Could you check a few things on this drawing? It's one solid part, dimensions in mm from its lowest x, y, z. A direction names the side the tool comes from. Give positions to 0.01 mm unless a question says otherwise; leave off trailing zeros. Loops run counter-clockwise (first coordinate to the right, second up) from the corner with the lowest first, then second, coordinate; pieces in that order, holes last. Notation, with made-up numbers: M -17,20.5 L 3,20.5 A22 ccw 3,37.5 Z; hole C 58.25,6.25 d3. An arc over 180 degrees is marked long. Answer as CSV lines item,"result". Start each with the question number.
Item 1: Will these pins go through, and if not, where does the flat tip stop? P1, Ø5, axis at x = 364.5, z = 446.5, coming from the +Y side; P2, Ø10, axis at x = 457.5, y = 46.5, coming from the +Z side; P3, Ø2, axis at y = 214.5, z = 768, coming from the -X side.
Item 2: I want a section at B-B on z = 184. List the corners of the cut face in (x, y) for me.
Item 3: If we mould it in two halves opening along Z, with no side actions, what happens to the marked faces 3, 4 and 5? For each: released by +Z, released by -Z, zero draft, split by the parting line, or undercut.
Item 4: If I drill on line 1 along Z through (x, y) = (636, 137.5); line 2 along X through (y, z) = (44.5, 794.5); line 3 along Z through (x, y) = (797.5, 50.5), over which ranges is the centre line in solid material (lowest first)? Write a range as from..to.
Item 5: I want a section at A-A on y = 223.5. List the corners of the cut face in (x, z) for me, plus the area to 3 significant figures.
Item 6: For the marked faces 1 and 2, which set-ups out of +Z, -Z, +X, -X, +Y, -Y let a thin tool reach every point of the face, with its end or its side?
Item 7: I want a section at C-C on x = 959. List the corners of the cut face in (y, z) for me, plus the area to 3 significant figures.
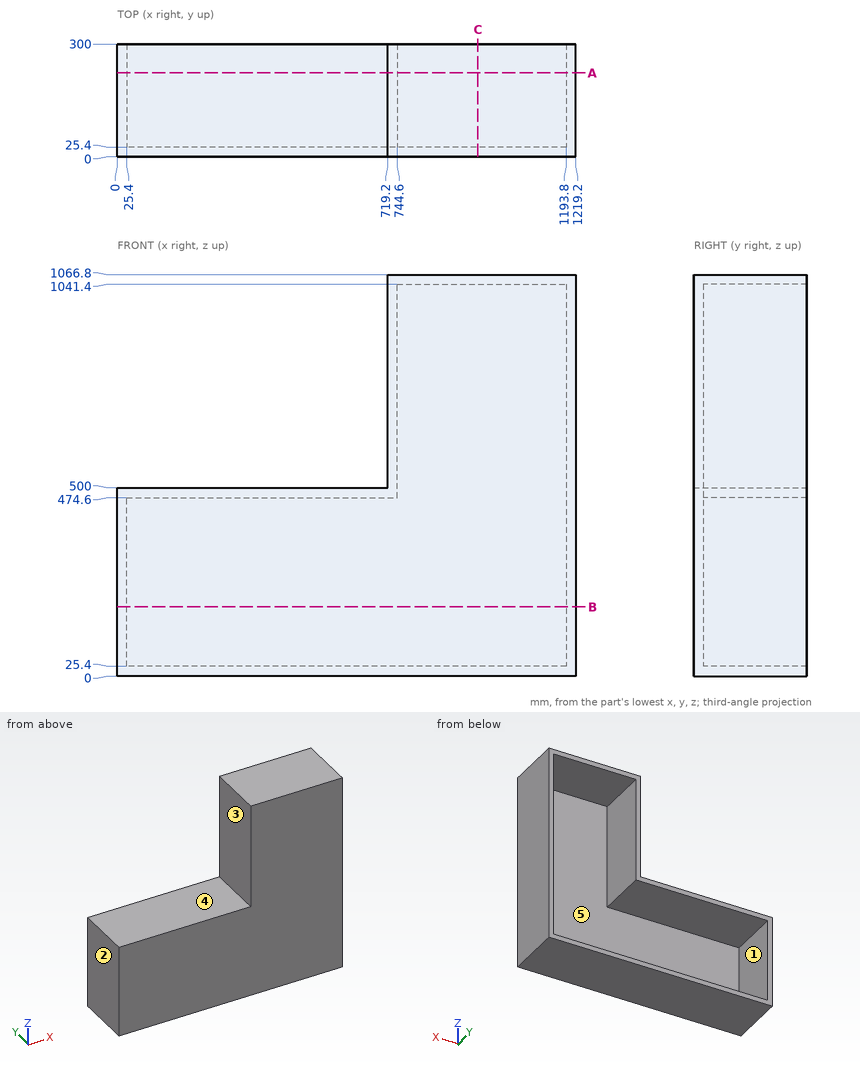
Result:
1,P1,"y = 25.4"
1,P2,"z = 500"
1,P3,"x = 719.2"
2,outline,"M 0,0 L 1219.2,0 L 1219.2,300 L 1193.8,300 L 1193.8,25.4 L 25.4,25.4 L 25.4,300 L 0,300 Z"
3,face 3,"zero draft"
3,face 4,"released by +Z"
3,face 5,"undercut"
4,line 1,"0..25.4, 474.6..500"
4,line 2,"719.2..744.6, 1193.8..1219.2"
4,line 3,"0..25.4, 1041.4..1066.8"
5,outline,"M 0,0 L 1219.2,0 L 1219.2,1066.8 L 719.2,1066.8 L 719.2,500 L 0,500 Z; hole M 25.4,25.4 L 1193.8,25.4 L 1193.8,1041.4 L 744.6,1041.4 L 744.6,474.6 L 25.4,474.6 Z"
5,area,"114,000 mm^2"
6,face 1,"+Y"
6,face 2,"+Z, -Z, -X, +Y, -Y"
7,outline,"M 0,0 L 300,0 L 300,25.4 L 25.4,25.4 L 25.4,1041.4 L 300,1041.4 L 300,1066.8 L 0,1066.8 Z"
7,area,"41,000 mm^2"
